from build123d import *

# Parameters (mm, degrees)
F0_R     = 1.6
F1_DEPTH = 3.175


# Not quite as in the source:
# - a length typed as a fraction of an inch, garbled in the dataset ("3 / 203.2 mm" for 3/8 in), is restored


with BuildPart() as f1:
    # F0 (on Front) → F1 (new body)
    with BuildSketch(Plane.XZ):
        with BuildLine():
            Line((47.46, 0), (2.54, 0))
            ThreePointArc((2.54, 0), (0.7439487758, -0.7439487758), (0, -2.54))
            Line((0, -2.54), (0, -77.46))
            ThreePointArc((0, -77.46), (0.7439487758, -79.2560512242), (2.54, -80))
            Line((2.54, -80), (47.46, -80))
            ThreePointArc((47.46, -80), (49.2560512242, -79.2560512242), (50, -77.46))
            Line((50, -77.46), (50, -2.54))
            ThreePointArc((50, -2.54), (49.2560512242, -0.7439487758), (47.46, 0))
        make_face()
        with Locations((5, -75)):
            Circle(F0_R, mode=Mode.SUBTRACT)
        with Locations((5, -65)):
            Circle(F0_R, mode=Mode.SUBTRACT)
        with Locations((15, -75)):
            Circle(F0_R, mode=Mode.SUBTRACT)
        with Locations((15, -65)):
            Circle(F0_R, mode=Mode.SUBTRACT)
        with Locations((5, -55)):
            Circle(F0_R, mode=Mode.SUBTRACT)
        with Locations((5, -45)):
            Circle(F0_R, mode=Mode.SUBTRACT)
        with Locations((15, -55)):
            Circle(F0_R, mode=Mode.SUBTRACT)
        with Locations((15, -45)):
            Circle(F0_R, mode=Mode.SUBTRACT)
        with Locations((25, -75)):
            Circle(F0_R, mode=Mode.SUBTRACT)
        with Locations((35, -75)):
            Circle(F0_R, mode=Mode.SUBTRACT)
        with Locations((25, -65)):
            Circle(F0_R, mode=Mode.SUBTRACT)
        with Locations((35, -65)):
            Circle(F0_R, mode=Mode.SUBTRACT)
        with Locations((45, -75)):
            Circle(F0_R, mode=Mode.SUBTRACT)
        with Locations((45, -65)):
            Circle(F0_R, mode=Mode.SUBTRACT)
        with Locations((25, -55)):
            Circle(F0_R, mode=Mode.SUBTRACT)
        with Locations((35, -55)):
            Circle(F0_R, mode=Mode.SUBTRACT)
        with Locations((25, -45)):
            Circle(F0_R, mode=Mode.SUBTRACT)
        with Locations((35, -45)):
            Circle(F0_R, mode=Mode.SUBTRACT)
        with Locations((45, -55)):
            Circle(F0_R, mode=Mode.SUBTRACT)
        with Locations((45, -45)):
            Circle(F0_R, mode=Mode.SUBTRACT)
        with Locations((5, -35)):
            Circle(F0_R, mode=Mode.SUBTRACT)
        with Locations((5, -25)):
            Circle(F0_R, mode=Mode.SUBTRACT)
        with Locations((15, -35)):
            Circle(F0_R, mode=Mode.SUBTRACT)
        with Locations((15, -25)):
            Circle(F0_R, mode=Mode.SUBTRACT)
        with Locations((5, -15)):
            Circle(F0_R, mode=Mode.SUBTRACT)
        with Locations((5, -5)):
            Circle(F0_R, mode=Mode.SUBTRACT)
        with Locations((15, -15)):
            Circle(F0_R, mode=Mode.SUBTRACT)
        with Locations((15, -5)):
            Circle(F0_R, mode=Mode.SUBTRACT)
        with Locations((25, -35)):
            Circle(F0_R, mode=Mode.SUBTRACT)
        with Locations((35, -35)):
            Circle(F0_R, mode=Mode.SUBTRACT)
        with Locations((25, -25)):
            Circle(F0_R, mode=Mode.SUBTRACT)
        with Locations((35, -25)):
            Circle(F0_R, mode=Mode.SUBTRACT)
        with Locations((45, -35)):
            Circle(F0_R, mode=Mode.SUBTRACT)
        with Locations((45, -25)):
            Circle(F0_R, mode=Mode.SUBTRACT)
        with Locations((25, -15)):
            Circle(F0_R, mode=Mode.SUBTRACT)
        with Locations((35, -15)):
            Circle(F0_R, mode=Mode.SUBTRACT)
        with Locations((25, -5)):
            Circle(F0_R, mode=Mode.SUBTRACT)
        with Locations((35, -5)):
            Circle(F0_R, mode=Mode.SUBTRACT)
        with Locations((45, -15)):
            Circle(F0_R, mode=Mode.SUBTRACT)
        with Locations((45, -5)):
            Circle(F0_R, mode=Mode.SUBTRACT)
    extrude(amount=F1_DEPTH)


solid = f1.part
Here's how the part is built. I have some questions about the finished solid (model axes, mm). Coordinates: 2 decimals unless noted, no trailing zeros. Loops run counter-clockwise (first coordinate to the right, second up) from the corner with the lowest first, then second, coordinate; pieces in that order, holes last.
1. Imagine slicing it at B-B, the plane y = -1.35. Count the separate pieces of the cut face and the enclosed holes in it, and give its area (3 significant figures).
2. I need wall thicknesses on L1, parallel to X at y = -1.2, z = -75; L2, parallel to X at y = -2.2, z = -14. Which ranges of each line are inside material? Lowest first, please.
3. Imagine slicing it at A-A, the plane z = -5. Please give me the cut outline in (x, y) (3 decimals).
4. If we mould it in two halves opening along Z, with no side actions, what happens to faces 1 (the flat face through (25, -2, -80)), 2 (the cylindrical face through (49.276, -1.565, -0.764)), 3 (the cylindrical face through (44.792, -1.565, -73.414))? For each: pulls with the +Z half, pulls with the -Z half, needs draft (parallel to the pull), parting line crosses it, or undercut.
Taken from the geometry:
1. separate pieces: 1
1. enclosed holes: 40
1. area: 3,670 mm2
2. L1: x = 0 to 3.4, 6.6 to 13.4, 16.6 to 23.4, 26.6 to 33.4, 36.6 to 43.4, 46.6 to 50
2. L2: x = 0 to 3.75, 6.25 to 13.75, 16.25 to 23.75, 26.25 to 33.75, 36.25 to 43.75, 46.25 to 50
3. outline: (0, -3.175) - (3.4, -3.175) - (3.4, 0) - (0, 0) - close; (6.6, -3.175) - (13.4, -3.175) - (13.4, 0) - (6.6, 0) - close; (16.6, -3.175) - (23.4, -3.175) - (23.4, 0) - (16.6, 0) - close; (26.6, -3.175) - (33.4, -3.175) - (33.4, 0) - (26.6, 0) - close; (36.6, -3.175) - (43.4, -3.175) - (43.4, 0) - (36.6, 0) - close; (46.6, -3.175) - (50, -3.175) - (50, 0) - (46.6, 0) - close
4. face 1: pulls with the -Z half
4. face 2: pulls with the +Z half
4. face 3: undercut
